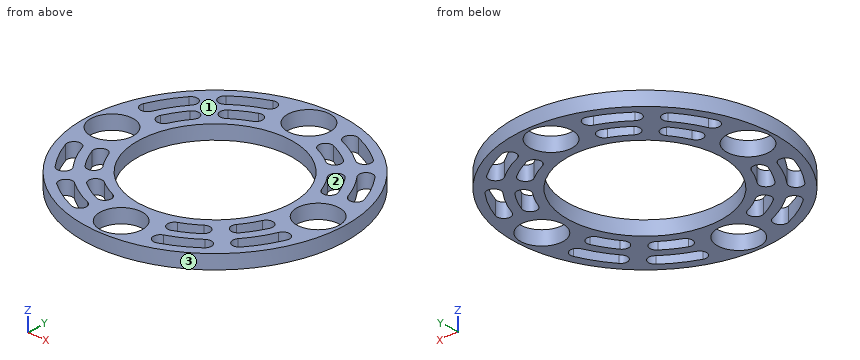
```python
from build123d import *

# Parameters (mm, degrees)
SKETCH6_R           = 58.75
SKETCH6_R_2         = 34.5
BOSS_EXTRUDE1_DEPTH = 6.35
SKETCH5_R           = 9.55
CUT_EXTRUDE1_DEPTH  = 7.35
CUT_EXTRUDE3_DEPTH  = 7.35


with BuildPart() as part:
    # Sketch6 → Boss-Extrude1 (new body)
    with BuildSketch(Plane.XY):
        Circle(SKETCH6_R)
        Circle(SKETCH6_R_2, mode=Mode.SUBTRACT)
    extrude(amount=BOSS_EXTRUDE1_DEPTH)

    # Sketch5 → Cut-Extrude1 (cut, through all)
    with BuildSketch(Plane.XY):
        with Locations((0, 47.6)):
            Circle(SKETCH5_R)
        with Locations((47.6, 0)):
            Circle(SKETCH5_R)
        with Locations((0, -47.6)):
            Circle(SKETCH5_R)
        with Locations((-47.6, 0)):
            Circle(SKETCH5_R)
    extrude(amount=CUT_EXTRUDE1_DEPTH, mode=Mode.SUBTRACT)

    # Sketch9 → Cut-Extrude3 (cut, through all)
    with BuildSketch(Plane.XY):
        with BuildLine():
            ThreePointArc((33.958355337, 42.946392198), (27.156576229, 47.540328854), (19.744469053, 51.065824597))
            ThreePointArc((19.744469053, 51.065824597), (15.783619294, 49.313830965), (17.535612926, 45.352981206))
            ThreePointArc((17.535612926, 45.352981206), (24.118511765, 42.221890237), (30.159361247, 38.141887135))
            ThreePointArc((30.159361247, 38.141887135), (34.461110824, 38.644642621), (33.958355337, 42.946392198))
        make_face()
        with BuildLine():
            ThreePointArc((51.065824597, 19.744469053), (47.540328854, 27.156576229), (42.946392198, 33.958355337))
            ThreePointArc((42.946392198, 33.958355337), (38.644642621, 34.461110824), (38.141887135, 30.159361247))
            ThreePointArc((38.141887135, 30.159361247), (42.221890237, 24.118511765), (45.352981206, 17.535612926))
            ThreePointArc((45.352981206, 17.535612926), (49.313830965, 15.783619294), (51.065824597, 19.744469053))
        make_face()
        with BuildLine():
            ThreePointArc((26.668852196, 35.779364829), (22.171350506, 38.72753338), (17.351873742, 41.113295935))
            ThreePointArc((17.351873742, 41.113295935), (13.339558176, 39.482610098), (14.970244012, 35.470294532))
            ThreePointArc((14.970244012, 35.470294532), (19.128223966, 33.411989583), (23.008421502, 30.868471617))
            ThreePointArc((23.008421502, 30.868471617), (27.294083455, 31.493702876), (26.668852196, 35.779364829))
        make_face()
        with BuildLine():
            ThreePointArc((41.113295935, 17.351873742), (38.72753338, 22.171350506), (35.779364829, 26.668852196))
            ThreePointArc((35.779364829, 26.668852196), (31.493702876, 27.294083455), (30.868471617, 23.008421502))
            ThreePointArc((30.868471617, 23.008421502), (33.411989583, 19.128223966), (35.470294532, 14.970244012))
            ThreePointArc((35.470294532, 14.970244012), (39.482610098, 13.339558176), (41.113295935, 17.351873742))
        make_face()
        with BuildLine():
            ThreePointArc((-33.958355337, 42.946392198), (-27.156576229, 47.540328854), (-19.744469053, 51.065824597))
            ThreePointArc((-19.744469053, 51.065824597), (-15.783619294, 49.313830965), (-17.535612926, 45.352981206))
            ThreePointArc((-17.535612926, 45.352981206), (-24.118511765, 42.221890237), (-30.159361247, 38.141887135))
            ThreePointArc((-30.159361247, 38.141887135), (-34.461110824, 38.644642621), (-33.958355337, 42.946392198))
        make_face()
        with BuildLine():
            ThreePointArc((-51.065824597, 19.744469053), (-47.540328854, 27.156576229), (-42.946392198, 33.958355337))
            ThreePointArc((-42.946392198, 33.958355337), (-38.644642621, 34.461110824), (-38.141887135, 30.159361247))
            ThreePointArc((-38.141887135, 30.159361247), (-42.221890237, 24.118511765), (-45.352981206, 17.535612926))
            ThreePointArc((-45.352981206, 17.535612926), (-49.313830965, 15.783619294), (-51.065824597, 19.744469053))
        make_face()
        with BuildLine():
            ThreePointArc((-26.668852196, 35.779364829), (-22.171350506, 38.72753338), (-17.351873742, 41.113295935))
            ThreePointArc((-17.351873742, 41.113295935), (-13.339558176, 39.482610098), (-14.970244012, 35.470294532))
            ThreePointArc((-14.970244012, 35.470294532), (-19.128223966, 33.411989583), (-23.008421502, 30.868471617))
            ThreePointArc((-23.008421502, 30.868471617), (-27.294083455, 31.493702876), (-26.668852196, 35.779364829))
        make_face()
        with BuildLine():
            ThreePointArc((-41.113295935, 17.351873742), (-38.72753338, 22.171350506), (-35.779364829, 26.668852196))
            ThreePointArc((-35.779364829, 26.668852196), (-31.493702876, 27.294083455), (-30.868471617, 23.008421502))
            ThreePointArc((-30.868471617, 23.008421502), (-33.411989583, 19.128223966), (-35.470294532, 14.970244012))
            ThreePointArc((-35.470294532, 14.970244012), (-39.482610098, 13.339558176), (-41.113295935, 17.351873742))
        make_face()
        with BuildLine():
            ThreePointArc((-33.958355337, -42.946392198), (-27.156576229, -47.540328854), (-19.744469053, -51.065824597))
            ThreePointArc((-19.744469053, -51.065824597), (-15.783619294, -49.313830965), (-17.535612926, -45.352981206))
            ThreePointArc((-17.535612926, -45.352981206), (-24.118511765, -42.221890237), (-30.159361247, -38.141887135))
            ThreePointArc((-30.159361247, -38.141887135), (-34.461110824, -38.644642621), (-33.958355337, -42.946392198))
        make_face()
        with BuildLine():
            ThreePointArc((-51.065824597, -19.744469053), (-47.540328854, -27.156576229), (-42.946392198, -33.958355337))
            ThreePointArc((-42.946392198, -33.958355337), (-38.644642621, -34.461110824), (-38.141887135, -30.159361247))
            ThreePointArc((-38.141887135, -30.159361247), (-42.221890237, -24.118511765), (-45.352981206, -17.535612926))
            ThreePointArc((-45.352981206, -17.535612926), (-49.313830965, -15.783619294), (-51.065824597, -19.744469053))
        make_face()
        with BuildLine():
            ThreePointArc((-26.668852196, -35.779364829), (-22.171350506, -38.72753338), (-17.351873742, -41.113295935))
            ThreePointArc((-17.351873742, -41.113295935), (-13.339558176, -39.482610098), (-14.970244012, -35.470294532))
            ThreePointArc((-14.970244012, -35.470294532), (-19.128223966, -33.411989583), (-23.008421502, -30.868471617))
            ThreePointArc((-23.008421502, -30.868471617), (-27.294083455, -31.493702876), (-26.668852196, -35.779364829))
        make_face()
        with BuildLine():
            ThreePointArc((-41.113295935, -17.351873742), (-38.72753338, -22.171350506), (-35.779364829, -26.668852196))
            ThreePointArc((-35.779364829, -26.668852196), (-31.493702876, -27.294083455), (-30.868471617, -23.008421502))
            ThreePointArc((-30.868471617, -23.008421502), (-33.411989583, -19.128223966), (-35.470294532, -14.970244012))
            ThreePointArc((-35.470294532, -14.970244012), (-39.482610098, -13.339558176), (-41.113295935, -17.351873742))
        make_face()
        with BuildLine():
            ThreePointArc((33.958355337, -42.946392198), (27.156576229, -47.540328854), (19.744469053, -51.065824597))
            ThreePointArc((19.744469053, -51.065824597), (15.783619294, -49.313830965), (17.535612926, -45.352981206))
            ThreePointArc((17.535612926, -45.352981206), (24.118511765, -42.221890237), (30.159361247, -38.141887135))
            ThreePointArc((30.159361247, -38.141887135), (34.461110824, -38.644642621), (33.958355337, -42.946392198))
        make_face()
        with BuildLine():
            ThreePointArc((26.668852196, -35.779364829), (22.171350506, -38.72753338), (17.351873742, -41.113295935))
            ThreePointArc((17.351873742, -41.113295935), (13.339558176, -39.482610098), (14.970244012, -35.470294532))
            ThreePointArc((14.970244012, -35.470294532), (19.128223966, -33.411989583), (23.008421502, -30.868471617))
            ThreePointArc((23.008421502, -30.868471617), (27.294083455, -31.493702876), (26.668852196, -35.779364829))
        make_face()
        with BuildLine():
            ThreePointArc((41.113295935, -17.351873742), (38.72753338, -22.171350506), (35.779364829, -26.668852196))
            ThreePointArc((35.779364829, -26.668852196), (31.493702876, -27.294083455), (30.868471617, -23.008421502))
            ThreePointArc((30.868471617, -23.008421502), (33.411989583, -19.128223966), (35.470294532, -14.970244012))
            ThreePointArc((35.470294532, -14.970244012), (39.482610098, -13.339558176), (41.113295935, -17.351873742))
        make_face()
        with BuildLine():
            ThreePointArc((51.065824597, -19.744469053), (47.540328854, -27.156576229), (42.946392198, -33.958355337))
            ThreePointArc((42.946392198, -33.958355337), (38.644642621, -34.461110824), (38.141887135, -30.159361247))
            ThreePointArc((38.141887135, -30.159361247), (42.221890237, -24.118511765), (45.352981206, -17.535612926))
            ThreePointArc((45.352981206, -17.535612926), (49.313830965, -15.783619294), (51.065824597, -19.744469053))
        make_face()
    extrude(amount=CUT_EXTRUDE3_DEPTH, mode=Mode.SUBTRACT)


solid = part.part
```
Build history of the part. All positions in model axes, mm. Face numbers are marked on the shaded views. Coordinates: 2 decimals unless noted, no trailing zeros. Order: outer loops, then holes, each group sorted by start corner. A loop starts at its lowest first (then second) coordinate and runs counter-clockwise, first axis right, second up. Notation, with made-up numbers: (19.5, 18.5) -> (37.5, 18.5) arc R32 ccw to (37.5, 52.5) -> close; hole circle Ø2 at (16.25, 66). An arc over 180 degrees is marked (long way). Answer in a Markdown table with one row per item. Add a question column.
Q1. Wall check: line 1 along Y through (x, z) = (0, 4.25); line 2 along Y through (x, z) = (20, 3.25); line 3 along Y through (x, z) = (6, 5.5). Give the ranges that are in metal, low to high. Write a range as [from, to].
Q2. Drop flat-ended pins along their axis: pin 1 (1.5 mm diameter, centred on x = 25, z = 3, fed in from +Y); pin 2 (2 mm diameter, centred on x = -3, z = 5.5, fed in from -Y); pin 3 (15.5 mm diameter, centred on x = 0, y = -47.6, fed in from -Z). Give the stop position or say it passes through.
Q3. Band-saw the part on D-D, the plane z = 1.5. Give the number of separate pieces and of enclosed holes in the cut face, then the cut area to 3 significant figures.
Q4. Mould opens along Y. For the marked faces 1, 2 and 3 say: +Y half, -Y half, draft (parallel to the pull), parting line (faces both ways), or undercut.
Q5. Band-saw the part on C-C, the plane x = 24.5. List the corners of the cut face in (y, z).
Q6. Band-saw the part on A-A, the plane y = 0. List the corners of the cut face in (x, z), then the cut area to 3 significant figures.
Answers follow:
| question | item | result |
|---|---|---|
| 1 | line 1 | [-58.75, -57.15], [-38.05, -34.5], [34.5, 38.05], [57.15, 58.75] |
| 1 | line 2 | [-55.24, -50.97], [-44.32, -39.89], [-32.9, -28.11], [28.11, 32.9], [39.89, 44.32], [50.97, 55.24] |
| 1 | line 3 | [-58.44, -55.03], [-40.17, -33.97], [33.97, 40.17], [55.03, 58.44] |
| 2 | pin 1 | y = 53.51 |
| 2 | pin 2 | y = -58.72 |
| 2 | pin 3 | through |
| 3 | separate pieces | 1 |
| 3 | enclosed holes | 21 |
| 3 | area | 4,240 mm^2 |
| 4 | face 1 | draft |
| 4 | face 2 | undercut |
| 4 | face 3 | parting line |
| 5 | outline | (-53.4, 0) -> (-48.96, 0) -> (-48.96, 6.35) -> (-53.4, 6.35) -> close; (-42, 0) -> (-37.3, 0) -> (-37.3, 6.35) -> (-42, 6.35) -> close; (-30.28, 0) -> (-24.29, 0) -> (-24.29, 6.35) -> (-30.28, 6.35) -> close; (24.29, 0) -> (30.28, 0) -> (30.28, 6.35) -> (24.29, 6.35) -> close; (37.3, 0) -> (42, 0) -> (42, 6.35) -> (37.3, 6.35) -> close; (48.96, 0) -> (53.4, 0) -> (53.4, 6.35) -> (48.96, 6.35) -> close |
| 6 | outline | (-58.75, 0) -> (-57.15, 0) -> (-57.15, 6.35) -> (-58.75, 6.35) -> close; (-38.05, 0) -> (-34.5, 0) -> (-34.5, 6.35) -> (-38.05, 6.35) -> close; (34.5, 0) -> (38.05, 0) -> (38.05, 6.35) -> (34.5, 6.35) -> close; (57.15, 0) -> (58.75, 0) -> (58.75, 6.35) -> (57.15, 6.35) -> close |
| 6 | area | 65.4 mm^2 |
